Can you work these out from the model? Positions are in its coordinate system, mm. Face numbers are marked on the shaded views. A direction names the side the tool comes from. Give positions to 0.01 mm unless a question says otherwise; leave off trailing zeros. Loops run counter-clockwise (first coordinate to the right, second up) from the corner with the lowest first, then second, coordinate; pieces in that order, holes last. Notation, with made-up numbers: (-35.75, 33.5) -> (-6.75, 33.5) arc R19 cw to (-6.75, 54.5) -> close; hole circle Ø1 at (3.5, 52). An arc over 180 degrees is marked (long way). One line per question, with ' | ' between items.
from build123d import *

# Parameters (mm, degrees)
SKETCH_1_W           = 80
SKETCH_1_H           = 60
EXTRUDE_1_DEPTH      = 5
SKETCH_2_R           = 1.75
SKETCH_2_R_2         = 11
CUT_EXTRUDE_1_DEPTH  = 51.249378106
SKETCH_3_W           = 36
SKETCH_3_H           = 60
EXTRUDE_2_DEPTH      = 15
SKETCH_4_R           = 4
SKETCH_4_W           = 25
SKETCH_4_H           = 10
CUT_EXTRUDE_7_DEPTH  = 57.885850613
EXTRUDE_6_DEPTH      = 22
SKETCH_15_R          = 7.5
CUT_EXTRUDE_8_DEPTH  = 85.876380696
SKETCH_16_R          = 5.1
CUT_EXTRUDE_9_DEPTH  = 87.02325267
FILLET_1_R           = 8
FILLET_2_R           = 5
FILLET_3_R           = 2
FILLET_4_R           = 2
SKETCH_20_R          = 1.75
CUT_EXTRUDE_11_DEPTH = 93.195444573
SKETCH_23_W          = 78
SKETCH_23_H          = 60
EXTRUDE_8_DEPTH      = 10
SKETCH_26_W          = 44
SKETCH_26_H          = 60
CUT_EXTRUDE_13_DEPTH = 10
EXTRUDE_9_DEPTH      = 5
FILLET_5_R           = 5
SKETCH_25_R          = 1.581789818
SKETCH_25_R_2        = 11
CUT_EXTRUDE_14_DEPTH = 83.097503007
CUT_EXTRUDE_15_DEPTH = 1.5
EXTRUDE_10_DEPTH     = 2
FILLET_6_R           = 1
CUT_EXTRUDE_16_DEPTH = 83.097503007
EXTRUDE_11_DEPTH     = 13.5


with BuildPart() as part:
    # 草图1 → 凸台-拉伸1 (new body)
    with BuildSketch(Plane(origin=(0, 0, 0), x_dir=(1, 0, 0), z_dir=(0, 1, 0))):
        Rectangle(SKETCH_1_W, SKETCH_1_H)
    extrude(amount=EXTRUDE_1_DEPTH)

    # 草图2 → 切除-拉伸1 (cut, through all)
    with BuildSketch(Plane(origin=(0, 5, 0), x_dir=(1, 0, 0), z_dir=(0, 1, 0))):
        with Locations(Location((-3, 15.5, 0), (0, 0, 270))):
            Circle(SKETCH_2_R)
        with Locations(Location((-3, -15.5, 0), (0, 0, 270))):
            Circle(SKETCH_2_R)
        with Locations(Location((-34, -15.5, 0), (0, 0, 270))):
            Circle(SKETCH_2_R)
        with Locations(Location((-34, 15.5, 0), (0, 0, 270))):
            Circle(SKETCH_2_R)
        with Locations(Location((-18.5, 0, 0), (0, 0, 270))):
            Circle(SKETCH_2_R_2)
    extrude(amount=-CUT_EXTRUDE_1_DEPTH, mode=Mode.SUBTRACT)

    # 草图3 → 凸台-拉伸2 (add)
    with BuildSketch(Plane(origin=(0, 5, 0), x_dir=(1, 0, 0), z_dir=(0, 1, 0))):
        with Locations((22, 0)):
            Rectangle(SKETCH_3_W, SKETCH_3_H)
    extrude(amount=EXTRUDE_2_DEPTH)

    # 草图4 → 切除-拉伸7 (cut, through all)
    with BuildSketch(Plane.ZY.offset(-4)):
        with Locations((-22.5, 12.5)):
            Circle(SKETCH_4_R)
        with Locations((22.5, 12.5)):
            Circle(SKETCH_4_R)
        with Locations((0, 12.5)):
            Rectangle(SKETCH_4_W, SKETCH_4_H)
    extrude(amount=-CUT_EXTRUDE_7_DEPTH, mode=Mode.SUBTRACT)

    # 草图14 → 凸台-拉伸6 (add)
    with BuildSketch(Plane(origin=(0, 20, 0), x_dir=(1, 0, 0), z_dir=(0, 1, 0))):
        Polygon((4, 30), (4, -18), (34, -18), (34, 20), (56, 20), (56, 30), align=None)
    extrude(amount=EXTRUDE_6_DEPTH)

    # 草图15 → 切除-拉伸8 (cut, through all)
    with BuildSketch(Plane.XY.offset(18)):
        with Locations((16.5, 31)):
            Circle(SKETCH_15_R)
    extrude(amount=-CUT_EXTRUDE_8_DEPTH, mode=Mode.SUBTRACT)

    # 草图16 → 切除-拉伸9 (cut, through all)
    with BuildSketch(Plane.XY.offset(-20)):
        with Locations((44.5, 31)):
            Circle(SKETCH_16_R)
    extrude(amount=-CUT_EXTRUDE_9_DEPTH, mode=Mode.SUBTRACT)

    # 圆角1
    fillet_1_edges = [part.edges().sort_by_distance(p)[0] for p in [
        (4, 42, -6),
    ]]
    fillet(fillet_1_edges, radius=FILLET_1_R)

    # 圆角2
    fillet_2_edges = [part.edges().sort_by_distance(p)[0] for p in [
        (34, 42, -1),
    ]]
    fillet(fillet_2_edges, radius=FILLET_2_R)

    # 圆角3
    fillet_3_edges = [part.edges().sort_by_distance(p)[0] for p in [
        (56, 42, -25),
    ]]
    fillet(fillet_3_edges, radius=FILLET_3_R)

    # 圆角4
    fillet_4_edges = [part.edges().sort_by_distance(p)[0] for p in [
        (40, 20, 5),
        (40, 0, 0),
        (56, 20, -25),
    ]]
    fillet(fillet_4_edges, radius=FILLET_4_R)

    # 草图20 → 切除-拉伸11 (cut, through all)
    with BuildSketch(Plane(origin=(0, 0, -30), x_dir=(-1, 0, 0), z_dir=(0, 0, -1))):
        with Locations((-44.135340411, 38.99168464)):
            Circle(SKETCH_20_R)
        with Locations((-36.50831536, 30.635340412)):
            Circle(SKETCH_20_R)
        with Locations((-44.864659589, 23.00831536)):
            Circle(SKETCH_20_R)
        with Locations((-52.49168464, 31.364659589)):
            Circle(SKETCH_20_R)
    extrude(amount=-CUT_EXTRUDE_11_DEPTH, mode=Mode.SUBTRACT)

    # 草图23 → 凸台-拉伸8 (add)
    with BuildSketch(Plane.XZ):
        with Locations((-1, 0)):
            Rectangle(SKETCH_23_W, SKETCH_23_H)
    extrude(amount=EXTRUDE_8_DEPTH)

    # 草图26 → 切除-拉伸13 (cut)
    with BuildSketch(Plane(origin=(0, 5, 0), x_dir=(1, 0, 0), z_dir=(0, 1, 0))):
        with Locations((-18, 0)):
            Rectangle(SKETCH_26_W, SKETCH_26_H)
    extrude(amount=-CUT_EXTRUDE_13_DEPTH, mode=Mode.SUBTRACT)

    # 草图29 → 凸台-拉伸9 (add)
    with BuildSketch(Plane.XY.offset(23)):
        Polygon((-40, -5), (-40, -21), (4, -37), (4, -5), align=None)
    extrude(amount=EXTRUDE_9_DEPTH)

    # 圆角5
    fillet_5_edges = [part.edges().sort_by_distance(p)[0] for p in [
        (38, -10, 0),
        (-40, -7.5, 30),
        (-40, -7.5, -30),
    ]]
    fillet(fillet_5_edges, radius=FILLET_5_R)

    # 草图25 → 切除-拉伸14 (cut, through all)
    with BuildSketch(Plane.XZ.offset(10)):
        with Locations(Location((-32.902220535, -12.494692857, 0), (0, 0, 270))):
            Circle(SKETCH_25_R)
        with Locations(Location((-1.902220535, 18.505307143, 0), (0, 0, 270))):
            Circle(SKETCH_25_R)
        with Locations(Location((-32.902220535, 18.505307143, 0), (0, 0, 270))):
            Circle(SKETCH_25_R)
        with Locations(Location((-1.902220535, -12.494692857, 0), (0, 0, 270))):
            Circle(SKETCH_25_R)
        with Locations(Location((-17.402220535, 3.005307143, 0), (0, 0, 270))):
            Circle(SKETCH_25_R_2)
    extrude(amount=-CUT_EXTRUDE_14_DEPTH, mode=Mode.SUBTRACT)

    # 草图30 → 切除-拉伸15 (cut)
    with BuildSketch(Plane(origin=(0, 0, 23), x_dir=(-1, 0, 0), z_dir=(0, 0, -1))):
        Polygon((-4, -10), (40, -10), (40, -21), (-4, -37), align=None)
    extrude(amount=-CUT_EXTRUDE_15_DEPTH, mode=Mode.SUBTRACT)

    # 草图31 → 凸台-拉伸10 (add)
    with BuildSketch(Plane.XY.offset(28)):
        Polygon((-39.701600618, -21.108508866), (-39.701600618, -10), (4, -10), (4, -37), align=None)
    extrude(amount=EXTRUDE_10_DEPTH)

    # 圆角6
    # the kernel refuses this fillet: 1 mm, written as the material it takes off along each edge
    with BuildSketch(Plane(origin=(-40, -10, 24.5), x_dir=(1, 0, 0), z_dir=(0, -1, 0))) as fillet_6_piece_1:
        with BuildLine():
            CenterArc((1.031373033, 1), FILLET_6_R, 172.819244219, 97.180755781)
            Line((0.039216292, 1.125), (-0.059999382, 1.1375))
            ThreePointArc((-0.059999382, 1.1375), (-0.1, 0.5), (-0.1, 0))
            Line((-0.1, 0), (0, -0.1))
            Line((0, -0.1), (1.031373033, -0.1))
            Line((1.031373033, -0.1), (1.031373033, 0))
        make_face()
    extrude(amount=13.814208278, mode=Mode.SUBTRACT)
    with BuildSketch(Plane(origin=(6.349483559, -37.854357658, 30), x_dir=(0.34174306308670427, 0.9397934234884371, 0), z_dir=(-0.9397934234884371, 0.3417430630867043, 0))) as fillet_6_piece_2:
        with BuildLine():
            CenterArc((FILLET_6_R, FILLET_6_R), FILLET_6_R, 180, 90)
            Line((0, FILLET_6_R), (-FILLET_6_R * 0.02, FILLET_6_R))
            Line((-FILLET_6_R * 0.02, FILLET_6_R), (-FILLET_6_R * 0.02, -FILLET_6_R * 0.02))
            Line((-FILLET_6_R * 0.02, -FILLET_6_R * 0.02), (FILLET_6_R, -FILLET_6_R * 0.02))
            Line((FILLET_6_R, -FILLET_6_R * 0.02), (FILLET_6_R, 0))
        make_face()
    extrude(amount=51.501283714, mode=Mode.SUBTRACT)
    with BuildSketch(Plane(origin=(-39.701600618, -23.49461161, 28), x_dir=(1, 0, 0), z_dir=(0, 1, 0))) as fillet_6_piece_3_section:
        with BuildLine():
            CenterArc((1, -0.954441098), FILLET_6_R, 107.361491651, 72.638508349)
            Line((0, -0.954441098), (-0.02, -0.954441098))
            Line((-0.02, -0.954441098), (-0.02, 0))
            Line((-0.02, 0), (0, 0.02))
            ThreePointArc((0, 0.02), (0.350800309, 0.02), (0.69563263, 0.019088822))
            Line((0.69563263, 0.019088822), (0.701600618, 0))
        make_face()
    fillet_6_piece_3 = extrude(amount=15.880714354, mode=Mode.PRIVATE)
    fillet_6_piece_3 = fillet_6_piece_3 - Plane(origin=(-35, -15.554254433, 25), x_dir=(0, 0, 1), z_dir=(0, -1, 0)) * Cylinder(5, 36, mode=Mode.PRIVATE)
    add(fillet_6_piece_3, mode=Mode.SUBTRACT)
    with BuildSketch(Plane(origin=(-39.701600618, -23.608508866, 30), x_dir=(1, 0, 0), z_dir=(0, 1, 0))) as fillet_6_piece_4:
        with BuildLine():
            CenterArc((FILLET_6_R, FILLET_6_R), FILLET_6_R, 180, 90)
            Line((0, FILLET_6_R), (-FILLET_6_R * 0.02, FILLET_6_R))
            Line((-FILLET_6_R * 0.02, FILLET_6_R), (-FILLET_6_R * 0.02, -FILLET_6_R * 0.02))
            Line((-FILLET_6_R * 0.02, -FILLET_6_R * 0.02), (FILLET_6_R, -FILLET_6_R * 0.02))
            Line((FILLET_6_R, -FILLET_6_R * 0.02), (FILLET_6_R, 0))
        make_face()
    extrude(amount=16.108508866, mode=Mode.SUBTRACT)

    # 草图32 → 切除-拉伸16 (cut, through all)
    with BuildSketch(Plane(origin=(0, -10, 0), x_dir=(1, 0, 0), z_dir=(0, 1, 0))):
        with BuildLine():
            Line((-39.701600618, -28.954441098), (-39.701600618, -29))
            ThreePointArc((-39.701600618, -29), (-39.408707399, -29.707106781), (-38.701600618, -30))
            Line((-38.701600618, -30), (-35, -30))
            ThreePointArc((-35, -30), (-37.236067977, -29.472135955), (-39, -28))
            ThreePointArc((-39, -28), (-39.507329909, -28.362157121), (-39.701600618, -28.954441098))
        make_face()
    extrude(amount=-CUT_EXTRUDE_16_DEPTH, mode=Mode.SUBTRACT)

    # 草图33 → 凸台-拉伸11 (add)
    with BuildSketch(Plane(origin=(4, 0, 0), x_dir=(0, 0, -1), z_dir=(1, 0, 0))):
        with BuildLine():
            Line((-30, -10), (-30, -35.935936372))
            add(Edge.make_bspline(
                [(-30, -35.935936372), (-30, -37), (-29, -37)],
                knots=[1.570796327, 1.570796327, 1.570796327, 3.141592654, 3.141592654, 3.141592654], degree=2, weights=[1, 0.707106781, 1]))
            Line((-29, -37), (-24.5, -37))
            Line((-24.5, -37), (-24.5, -10))
            Line((-24.5, -10), (-30, -10))
        make_face()
    extrude(amount=EXTRUDE_11_DEPTH)


solid = part.part
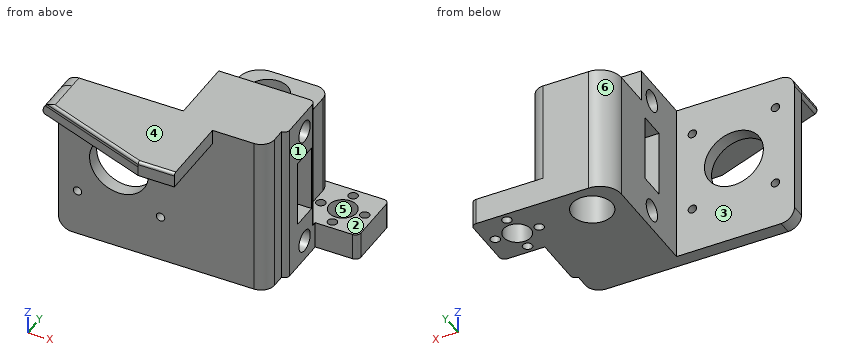
Q1. If I drill on probe 1 along Y at (x, z) = (15.5, -5); probe 2 along Z at (x, y) = (24.5, 10); probe 3 along Y at (x, z) = (11.5, 0), over which ranges is the centre line in solid material (lowest first)? Write a range as from..to.
Entries:
probe 1: -10..7.5, 17.5..23.57, 38.43..42 | probe 2: -30..-25.62, -19.38..-12.5, 12.5..19.38, 25.62..30 | probe 3: -10..7.5, 17.5..25.41, 36.59..41.98
Q2. For pin 1 Ø1 at (y, z) = (-3, 5.5) entering from -X; pin 2 Ø11 at (x, z) = (49, -26) entering from -Y; pin 3 Ø3.5 at (x, z) = (-1.9, 18.51) entering from -Y, each with a flat end and sliding along its axis, tell me the tip position at first contact or that it passes through.
Entries:
pin 1: x = 4 | pin 2: y = 20 | pin 3: y = -10
Q3. If we section it at D-D (z = 7.5): Write out the boundary of the cut face in (x, y).
Entries:
outline: (-40, -10) -> (-27.44, -10) -> (-27.44, -5) -> (-40, -5) -> close; (-7.36, -10) -> (33, -10) arc R5 ccw to (38, -5) -> (38, 0) arc R2 ccw to (40, 2) -> (40, 7.5) -> (4, 7.5) -> (4, -5) -> (-7.36, -5) -> close; (4, 17.5) -> (40, 17.5) -> (40, 18) arc R2 ccw to (38, 20) -> (34, 20) -> (34, 37) arc R5 ccw to (29, 42) -> (12, 42) arc R8 ccw to (4, 34) -> close; hole circle Ø15 at (16.5, 31)
Q4. If we section it at A-A (x = 19.5): Write out the boundary of the cut face in (y, z).
Entries:
outline: (-10, -30) -> (24.13, -30) -> (24.13, 18) -> (20, 18) -> (20, 30) -> (-10, 30) -> close; (37.87, -30) -> (42, -30) -> (42, 18) -> (37.87, 18) -> close; hole (7.5, -12.5) -> (17.5, -12.5) -> (17.5, 12.5) -> (7.5, 12.5) -> close; hole circle Ø8 at (12.5, -22.5); hole circle Ø8 at (12.5, 22.5)
Q5. If we mould it in two halves opening along X, with no side actions, what happens to the marked faces 4, 5 and 6? For each: pulls with the +X half, pulls with the -X half, needs draft (parallel to the pull), parting line crosses it, or undercut.
Entries:
face 4: needs draft | face 5: undercut | face 6: pulls with the -X half
Q6. On a 3-axis mill with a long thin cutter (end or side, diameter ignored), from which of +Z, -Z, +X, -X, +Y, -Y can I reach the whole of each face in a straight line? I mean the marked faces 1, 2 and 3. Say none if no direction works.
Entries:
face 1: +Z, -Z, +X, -Y | face 2: +Z, +X, +Y | face 3: +Z, -Z, -X, +Y
Q7. If we section it at B-B (z = -22.5): Write out the boundary of the cut face in (x, y).
Entries:
outline: (-40, -10) -> (33, -10) arc R5 ccw to (38, -5) -> (38, 0) arc R2 ccw to (40, 2) -> (40, 8.5) -> (4, 8.5) -> (4, -5) -> (-40, -5) -> close; (4, 16.5) -> (40, 16.5) -> (40, 20) -> (54, 20) arc R2 ccw to (56, 22) -> (56, 40) arc R2 ccw to (54, 42) -> (12, 42) arc R8 ccw to (4, 34) -> close; hole circle Ø15 at (16.5, 31); hole circle Ø3.5 at (36.51, 30.64); hole circle Ø10.2 at (44.5, 31); hole circle Ø3.5 at (44.14, 38.99); hole circle Ø3.5 at (44.86, 23.01); hole circle Ø3.5 at (52.49, 31.36)
Q8. If we section it at C-C (y = 12.5): Write out the boundary of the cut face in (x, z).
Entries:
outline: (4, -30) -> (40, -30) -> (40, -26.5) -> (4, -26.5) -> close; (4, -18.5) -> (40, -18.5) -> (40, -12.5) -> (4, -12.5) -> close; (4, 12.5) -> (40, 12.5) -> (40, 18.5) -> (4, 18.5) -> close; (4, 26.5) -> (40, 26.5) -> (40, 30) -> (4, 30) -> close
